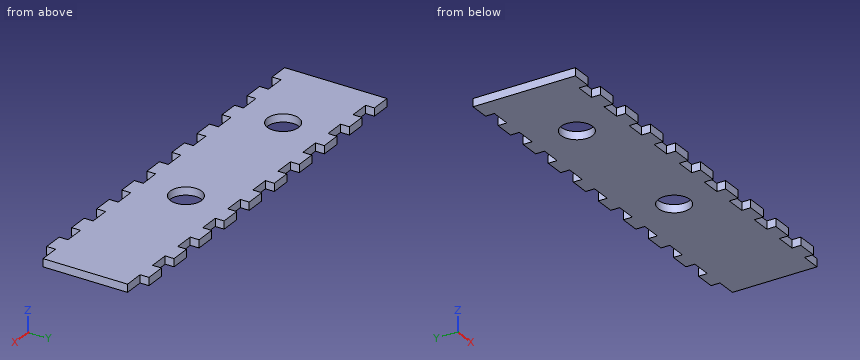
```python
from build123d import *

# Parameters (mm, degrees)
BOSS_EXTRUDE2_DEPTH = 2
SKETCH1_6_W         = 5
SKETCH1_6_H         = 2.25
BOSS_EXTRUDE4_DEPTH = 2


with BuildPart() as part:
    # Sketch1 → Boss-Extrude2 (new body)
    with BuildSketch(Plane.XY):
        with BuildLine():
            ThreePointArc((55.869934973, 10.7), (59.844934973, 14.675), (63.819934973, 10.7))
            Line((63.819934973, 10.7), (100, 10.7))
            Line((100, 10.7), (100, 21.4))
            Line((100, 21.4), (95, 21.4))
            Line((95, 21.4), (90, 21.4))
            Line((90, 21.4), (85, 21.4))
            Line((85, 21.4), (80, 21.4))
            Line((80, 21.4), (75, 21.4))
            Line((75, 21.4), (70, 21.4))
            Line((70, 21.4), (65, 21.4))
            Line((65, 21.4), (60, 21.4))
            Line((60, 21.4), (55, 21.4))
            Line((55, 21.4), (50, 21.4))
            Line((50, 21.4), (45, 21.4))
            Line((45, 21.4), (40, 21.4))
            Line((40, 21.4), (35, 21.4))
            Line((35, 21.4), (30, 21.4))
            Line((30, 21.4), (25, 21.4))
            Line((25, 21.4), (20, 21.4))
            Line((20, 21.4), (15, 21.4))
            Line((15, 21.4), (10, 21.4))
            Line((10, 21.4), (5, 21.4))
            Line((5, 21.4), (0, 21.4))
            Line((0, 21.4), (0, 10.7))
            Line((0, 10.7), (17.059934973, 10.7))
            ThreePointArc((17.059934973, 10.7), (21.034934973, 14.675), (25.009934973, 10.7))
            Line((25.009934973, 10.7), (55.869934973, 10.7))
        make_face()
        with BuildLine():
            Line((100, 10.7), (63.819934973, 10.7))
            ThreePointArc((63.819934973, 10.7), (59.844934973, 6.725), (55.869934973, 10.7))
            Line((55.869934973, 10.7), (25.009934973, 10.7))
            ThreePointArc((25.009934973, 10.7), (21.034934973, 6.725), (17.059934973, 10.7))
            Line((17.059934973, 10.7), (0, 10.7))
            Line((0, 10.7), (0, 0))
            Line((0, 0), (5, 0))
            Line((5, 0), (10, 0))
            Line((10, 0), (15, 0))
            Line((15, 0), (20, 0))
            Line((20, 0), (25, 0))
            Line((25, 0), (30, 0))
            Line((30, 0), (35, 0))
            Line((35, 0), (40, 0))
            Line((40, 0), (45, 0))
            Line((45, 0), (50, 0))
            Line((50, 0), (55, 0))
            Line((55, 0), (60, 0))
            Line((60, 0), (65, 0))
            Line((65, 0), (70, 0))
            Line((70, 0), (75, 0))
            Line((75, 0), (80, 0))
            Line((80, 0), (85, 0))
            Line((85, 0), (90, 0))
            Line((90, 0), (95, 0))
            Line((95, 0), (100, 0))
            Line((100, 0), (100, 10.7))
        make_face()
    extrude(amount=BOSS_EXTRUDE2_DEPTH)

    # Sketch1_6 → Boss-Extrude4 (add)
    with BuildSketch(Plane.XY):
        with Locations((2.5, -1.125)):
            Rectangle(SKETCH1_6_W, SKETCH1_6_H)
        with Locations((12.5, -1.125)):
            Rectangle(SKETCH1_6_W, SKETCH1_6_H)
        with Locations((92.5, -1.125)):
            Rectangle(SKETCH1_6_W, SKETCH1_6_H)
        with Locations((82.5, -1.125)):
            Rectangle(SKETCH1_6_W, SKETCH1_6_H)
        with Locations((72.5, -1.125)):
            Rectangle(SKETCH1_6_W, SKETCH1_6_H)
        with Locations((22.5, -1.125)):
            Rectangle(SKETCH1_6_W, SKETCH1_6_H)
        with Locations((32.5, -1.125)):
            Rectangle(SKETCH1_6_W, SKETCH1_6_H)
        with Locations((42.5, -1.125)):
            Rectangle(SKETCH1_6_W, SKETCH1_6_H)
        with Locations((52.5, -1.125)):
            Rectangle(SKETCH1_6_W, SKETCH1_6_H)
        with Locations((62.5, -1.125)):
            Rectangle(SKETCH1_6_W, SKETCH1_6_H)
        with Locations((2.5, 22.525)):
            Rectangle(SKETCH1_6_W, SKETCH1_6_H)
        with Locations((12.5, 22.525)):
            Rectangle(SKETCH1_6_W, SKETCH1_6_H)
        with Locations((22.5, 22.525)):
            Rectangle(SKETCH1_6_W, SKETCH1_6_H)
        with Locations((32.5, 22.525)):
            Rectangle(SKETCH1_6_W, SKETCH1_6_H)
        with Locations((42.5, 22.525)):
            Rectangle(SKETCH1_6_W, SKETCH1_6_H)
        with Locations((52.5, 22.525)):
            Rectangle(SKETCH1_6_W, SKETCH1_6_H)
        with Locations((62.5, 22.525)):
            Rectangle(SKETCH1_6_W, SKETCH1_6_H)
        with Locations((72.5, 22.525)):
            Rectangle(SKETCH1_6_W, SKETCH1_6_H)
        with Locations((92.5, 22.525)):
            Rectangle(SKETCH1_6_W, SKETCH1_6_H)
        with Locations((82.5, 22.525)):
            Rectangle(SKETCH1_6_W, SKETCH1_6_H)
    extrude(amount=BOSS_EXTRUDE4_DEPTH)


solid = part.part
```
The listing builds one solid part. Answer for the finished solid, in the listing's coordinates (mm). Coordinates: 2 decimals unless noted, no trailing zeros. Write each loop counter-clockwise with the first axis right and the second up, starting at its lowest first coordinate (ties: lowest second). Pieces come first, ordered by that corner, then holes. Notation, with made-up numbers: M -4,-1.75 L 39,-1.75 A13 cw 39,7.25 Z; hole C -14,48 d9. An arc over 180 degrees is marked long. Use a Markdown table: item, result. Add a question column.
1. Section B-B (x = 23.5) is taken. Give the vertices of the cut face in (y, z), plus the area to 3 significant figures.
2. Section A-A (y = 10.7) is taken. Give the vertices of the cut face in (x, z), plus the area to 3 significant figures.
3. Given P1, Ø0.6, axis at y = 22.5, z = 0.5, coming from the +X side; P2, Ø0.6, axis at x = 7.5, z = 1.5, coming from the -Y side; P3, Ø12, axis at x = 18, y = 6, coming from the -Z side; P4, Ø6.5, axis at x = 21.03, y = 10.7, coming from the +Z side, each flat-ended and moving along its own axis, determine where each tip first touches the part or whether it passes through.
4. Section C-C (z = 1.65) is taken. Count the separate pieces of the cut face and the enclosed holes in it, plus the area to 3 significant figures.
5. Section D-D (x = 68) is taken. Give the vertices of the cut face in (y, z), plus the area to 3 significant figures.
6. Straight lines are drawn through the part: line 1 along X through (y, z) = (10.7, 0.55); line 2 along X through (y, z) = (13.5, 0.45); line 3 along Y through (x, z) = (48.5, 0.6). For each, find the intervals that lie inside material, in ascending order. Write a range as [from, to].
Data:
| question | item | result |
|---|---|---|
| 1 | outline | M -2.25,0 L 7.58,0 L 7.58,2 L -2.25,2 Z; M 13.82,0 L 23.65,0 L 23.65,2 L 13.82,2 Z |
| 1 | area | 39.3 mm2 |
| 2 | outline | M 0,0 L 17.06,0 L 17.06,2 L 0,2 Z; M 25.01,0 L 55.87,0 L 55.87,2 L 25.01,2 Z; M 63.82,0 L 100,0 L 100,2 L 63.82,2 Z |
| 2 | area | 168 mm2 |
| 3 | P1 | stops at x = 95 |
| 3 | P2 | stops at y = 0 |
| 3 | P3 | stops at z = 0 |
| 3 | P4 | passes through |
| 4 | separate pieces | 1 |
| 4 | enclosed holes | 2 |
| 4 | area | 2,270 mm2 |
| 5 | outline | M 0,0 L 21.4,0 L 21.4,2 L 0,2 Z |
| 5 | area | 42.8 mm2 |
| 6 | line 1 | x = [0, 17.06], [25.01, 55.87], [63.82, 100] |
| 6 | line 2 | x = [0, 18.21], [23.86, 57.02], [62.67, 100] |
| 6 | line 3 | y = [0, 21.4] |
